from build123d import *

# Parameters (mm, degrees)
P_IDAT_VYSUNUT_M1_DEPTH   = 4.999999888
ODEBRAT_VYSUNUT_M1_DEPTH  = 84.910666461
SKICA3_W                  = 16.00000076
SKICA3_H                  = 5.000002682
P_IDAT_VYSUNUT_M2_DEPTH   = 20
ODEBRAT_VYSUNUT_M3_DEPTH  = 87.116200856
ODEBRAT_VYSUNUT_M4_DEPTH  = 87.116200856
ODEBRAT_VYSUNUT_M5_DEPTH  = 87.116200856
ODEBRAT_VYSUNUT_M6_DEPTH  = 87.116200856
ZKOSEN_1_SIZE             = 4.000000656
ZKOSEN_2_SIZE             = 4.999998957
ZKOSEN_2_SIZE_2           = 4.999999888
ZKOSEN_3_SIZE             = 3.999999976
ZKOSEN_3_SIZE2            = 4.000000587
SKICA11_R                 = 1.7
ODEBRAT_VYSUNUT_M9_DEPTH  = 10
SKICA12_W                 = 16.00000076
SKICA12_H                 = 5.000002682
P_IDAT_VYSUNUT_M3_DEPTH   = 9
SKICA10_R                 = 1.6
SKICA10_R_2               = 1.599999993
ODEBRAT_VYSUNUT_M10_DEPTH = 9


with BuildPart() as part:
    # Skica1 → Přidat vysunutím1 (new body)
    with BuildSketch(Plane.XY.offset(4.999999888)):
        Polygon((45.999998971, 70.000000298), (-29.500000179, 70.000000298), (-29.500000179, 6.8e-07), (9.999999776, 6.8e-07), (45.999998971, 64.999998915), align=None)
    extrude(amount=-P_IDAT_VYSUNUT_M1_DEPTH)

    # Skica2 → Odebrat vysunutím1 (cut, through all)
    with BuildSketch(Plane.XY.offset(4.999999888)):
        Polygon((25.833334774, 59.999998659), (30.000000641, 64.999996523), (30.000000641, 70.000000298), (-29.500000179, 70.000000298), (-29.500000179, 41.000001132), (9.999999776, 41.000001132), align=None)
    extrude(amount=-ODEBRAT_VYSUNUT_M1_DEPTH, mode=Mode.SUBTRACT)

    # Skica3 → Přidat vysunutím2 (add)
    with BuildSketch(Plane.XY.offset(4.999999888)):
        with Locations((37.999999709, 67.499998957)):
            Rectangle(SKICA3_W, SKICA3_H)
    extrude(amount=P_IDAT_VYSUNUT_M2_DEPTH)

    # Skica5 → Odebrat vysunutím3 (cut, through all)
    with BuildSketch(Plane.XY.offset(4.999999888)):
        Polygon((-23.097474128, 4.468092229), (-23.010937497, 4.819194786), (-23.010937497, 5.180804525), (-23.097474128, 5.531907082), (-23.265523836, 5.85209718), (-23.505315185, 6.122766063), (-23.802915588, 6.328184158), (-24.141026661, 6.456412841), (-24.499999359, 6.500000134), (-24.85897392, 6.456412841), (-25.197084993, 6.328184158), (-25.494683534, 6.122766063), (-25.734476745, 5.85209718), (-25.90252459, 5.531907082), (-25.989063084, 5.180804525), (-25.989063084, 4.819194786), (-25.90252459, 4.468092229), (-25.734476745, 4.147903062), (-25.494683534, 3.877233714), (-25.197084993, 3.671815852), (-24.85897392, 3.543587169), (-24.499999359, 3.500000108), (-24.141026661, 3.543587169), (-23.802915588, 3.671815852), (-23.505315185, 3.877233714), (-23.265523836, 4.147903062), align=None)
    extrude(amount=-ODEBRAT_VYSUNUT_M3_DEPTH, mode=Mode.SUBTRACT)

    # Skica6 → Odebrat vysunutím4 (cut, through all)
    with BuildSketch(Plane.XY.offset(4.999999888)):
        Polygon((5.505315959, 3.877233714), (5.802914966, 3.671815852), (6.141026504, 3.543587169), (6.500000134, 3.500000108), (6.858973298, 3.543587169), (7.197084371, 3.671815852), (7.494683843, 3.877233714), (7.734475657, 4.147903062), (7.902524434, 4.468092229), (7.989062928, 4.819194786), (7.989062928, 5.180804525), (7.902524434, 5.531907082), (7.734475657, 5.85209718), (7.494683843, 6.122766063), (7.197084371, 6.328184158), (6.858973298, 6.456412841), (6.500000134, 6.500000134), (6.141026504, 6.456412841), (5.802914966, 6.328184158), (5.505315959, 6.122766063), (5.26552368, 5.85209718), (5.097475369, 5.531907082), (5.010936875, 5.180804525), (5.010936875, 4.819194786), (5.097475369, 4.468092229), (5.26552368, 4.147903062), align=None)
    extrude(amount=-ODEBRAT_VYSUNUT_M4_DEPTH, mode=Mode.SUBTRACT)

    # Skica7 → Odebrat vysunutím5 (cut, through all)
    with BuildSketch(Plane.XY.offset(4.999999888)):
        Polygon((-23.377234116, 35.005312413), (-23.171816021, 35.302914679), (-23.043585941, 35.641025752), (-23.000000045, 35.99999845), (-23.043585941, 36.358974874), (-23.171816021, 36.697082222), (-23.377234116, 36.994680762), (-23.647902533, 37.234473974), (-23.968091235, 37.402521819), (-24.319194257, 37.489064038), (-24.680804461, 37.489064038), (-25.031907484, 37.402521819), (-25.352096185, 37.234473974), (-25.622766465, 36.994680762), (-25.82818456, 36.697082222), (-25.956412777, 36.358974874), (-26.000000536, 35.99999845), (-25.956412777, 35.641025752), (-25.82818456, 35.302914679), (-25.622766465, 35.005312413), (-25.352096185, 34.765522927), (-25.031907484, 34.597471356), (-24.680804461, 34.510936588), (-24.319194257, 34.510936588), (-23.968091235, 34.597471356), (-23.647902533, 34.765522927), align=None)
    extrude(amount=-ODEBRAT_VYSUNUT_M5_DEPTH, mode=Mode.SUBTRACT)

    # Skica8 → Odebrat vysunutím6 (cut, through all)
    with BuildSketch(Plane.XY.offset(4.999999888)):
        Polygon((5.968092475, 34.597471356), (6.319194566, 34.510936588), (6.68080477, 34.510936588), (7.031906862, 34.597471356), (7.35209696, 34.765522927), (7.622765843, 35.005312413), (7.828184403, 35.302914679), (7.956412621, 35.641025752), (8.00000038, 35.99999845), (7.956412621, 36.358974874), (7.828184403, 36.697082222), (7.622765843, 36.994680762), (7.35209696, 37.234473974), (7.031906862, 37.402521819), (6.68080477, 37.489064038), (6.319194566, 37.489064038), (5.968092475, 37.402521819), (5.647902843, 37.234473974), (5.377233494, 36.994680762), (5.171815865, 36.697082222), (5.043587182, 36.358974874), (4.999999888, 35.99999845), (5.043587182, 35.641025752), (5.171815865, 35.302914679), (5.377233494, 35.005312413), (5.647902843, 34.765522927), align=None)
    extrude(amount=-ODEBRAT_VYSUNUT_M6_DEPTH, mode=Mode.SUBTRACT)

    # Zkosení1
    zkosen_1_edges = [part.edges().sort_by_distance(p)[0] for p in [
        (-29.500000179, 41.000001132, 2.499999944),
    ]]
    chamfer(zkosen_1_edges, length=ZKOSEN_1_SIZE)

    # Zkosení2
    # the kernel refuses this chamfer: 4.999999888, 4.999998957 mm, written as the material it adds along each edge
    with BuildSketch(Plane(origin=(58.858412936, 64.999997616, 4.999999888), x_dir=(0, -0.999621916702082, -0.027495884216655726), z_dir=(-1, 0, 0))) as zkosen_2_piece_1_section:
        Polygon((ZKOSEN_2_SIZE * 0.999621916686, ZKOSEN_2_SIZE * 0.0274958842162), (-ZKOSEN_2_SIZE_2 * 0.027495884218, ZKOSEN_2_SIZE_2 * 0.99962191675), (0, 0), align=None)
    zkosen_2_piece_1 = extrude(amount=41.716826979, mode=Mode.PRIVATE)
    zkosen_2_piece_1 = split(zkosen_2_piece_1, bisect_by=Plane(origin=(43.332283636, 60.183290695, 6.69217666), z_dir=(-0.8747913551064548, 0.4844998297533371, 0)), keep=Keep.TOP, mode=Mode.PRIVATE)
    zkosen_2_piece_1 = split(zkosen_2_piece_1, bisect_by=Plane(origin=(32.300745654, 67.760889889, 6.69217666), z_dir=(0.7682212055202173, -0.6401844885570597, 0)), keep=Keep.TOP, mode=Mode.PRIVATE)
    add(zkosen_2_piece_1)

    # Zkosení3
    zkosen_3_edges = [part.edges().sort_by_distance(p)[0] for p in [
        (-29.500000179, 6.8e-07, 2.499999944),
    ]]
    zkosen_3_side = [part.faces().sort_by_distance(p)[0] for p in [
        (-9.750000201, 6.8e-07, 2.499999944),
    ]]
    chamfer(zkosen_3_edges, length=ZKOSEN_3_SIZE, length2=ZKOSEN_3_SIZE2, reference=zkosen_3_side[0])

    # Skica11 → Odebrat vysunutím9 (cut)
    with BuildSketch(Plane(origin=(0, 0, 0), x_dir=(-1, 0, 0), z_dir=(0, 0, -1))):
        with Locations((-6.500000134, 35.99999845)):
            Circle(SKICA11_R)
        with Locations((24.499998894, 35.99999845)):
            Circle(SKICA11_R)
        with Locations((-6.500000134, 4.999999655)):
            Circle(SKICA11_R)
        with Locations((24.499999359, 4.999999655)):
            Circle(SKICA11_R)
    extrude(amount=-ODEBRAT_VYSUNUT_M9_DEPTH, mode=Mode.SUBTRACT)

    # Skica12 → Přidat vysunutím3 (add)
    with BuildSketch(Plane.XY.offset(24.999999888)):
        with Locations((37.999999709, 67.499998957)):
            Rectangle(SKICA12_W, SKICA12_H)
    extrude(amount=P_IDAT_VYSUNUT_M3_DEPTH)

    # Skica10 → Odebrat vysunutím10 (cut)
    with BuildSketch(Plane.XZ.offset(-64.999997616)):
        with Locations(Location((32.999999717, 21.999999776, 0), (0, 0, 270))):
            Circle(SKICA10_R)
        with Locations(Location((42.999999717, 21.999999776, 0), (0, 0, 270))):
            Circle(SKICA10_R_2)
    extrude(amount=-ODEBRAT_VYSUNUT_M10_DEPTH, mode=Mode.SUBTRACT)


solid = part.part
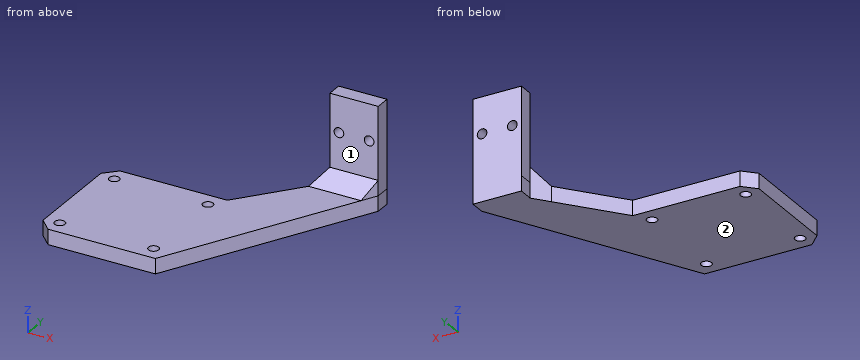
The listing builds one solid part. Answer for the finished solid, in the listing's coordinates (mm). Face numbers are marked on the shaded views. A direction names the side the tool comes from. Round coordinates to 2 decimals unless told otherwise and drop trailing zeros. Write each loop counter-clockwise with the first axis right and the second up, starting at its lowest first coordinate (ties: lowest second). Pieces come first, ordered by that corner, then holes. Notation, with made-up numbers: M 79,42.25 L 86,42.25 A19 cw 86,61.25 Z; hole C -38,80 d2. An arc over 180 degrees is marked long. Write each question's results on one line, items separated by ' | '. Start each with the question number.
(1) The part is cut by section B-B, the plane x = -24.5. Write down the section's boundary in (y, z), and give its area (3 significant figures).
(2) The part is cut by section C-C, the plane z = 4. Write down the section's boundary in (x, y).
(3) For the marked faces 1 and 2, determine the directions among +Z, -Z, +X, -X, +Y, -Y from which every point of the face is accessible in a straight line to the end or side of a thin tool.
(4) Find the intervals of material crossed by line 1 (X direction, y = 67, z = 22); line 2 (Y direction, x = 6.5, z = 2.8); line 3 (Z direction, x = 43, y = 67.55), in increasing order.
(5) The part is cut by section D-D, the plane x = 33. Write down the section's boundary in (y, z).
(6) The part is cut by section A-A, the plane z = 22. Write down the section's boundary in (x, y), and give its area (3 significant figures).
(7) Each of these flat-tipped pins is pushed along its axis until it touches: P1, Ø5.5, axis at y = 66.5, z = 16, coming from the -X side; P2, Ø5.5, axis at x = -4, z = 2.5, coming from the +Y side; P3, Ø2.5, axis at x = 33, z = 22, coming from the +Y side; P4, Ø2, axis at x = 1, y = 11.5, coming from the -Z side. Where does it stop, or does it pass through?
Worked answers:
1) outline: M 0,0 L 3.3,0 L 3.3,5 L 0,5 Z; M 6.7,0 L 34.3,0 L 34.3,5 L 6.7,5 Z; M 37.7,0 L 41,0 L 41,5 L 37.7,5 Z | area: 171 mm²
2) outline: M -29.5,4 L -25.5,0 L 10,0 L 46,65 L 46,70 L 30,70 L 30,65 L 10,41 L -25.5,41 L -29.5,37 Z; hole C -24.5,5 d3.4; hole C -24.5,36 d3.4; hole C 6.5,5 d3.4; hole C 6.5,36 d3.4
3) face 1: +Z, +X, -X, -Y | face 2: -Z, +X, -X, +Y, -Y
4) line 1: x = 30 to 31.4, 34.6 to 41.4, 44.6 to 46 | line 2: y = 0 to 3.3, 6.7 to 34.3, 37.7 to 41 | line 3: z = 0 to 20.4, 23.6 to 34
5) outline: M 41.53,0 L 70,0 L 70,20.4 L 65,20.4 L 65,10 L 60,5 L 41.53,5 Z; M 65,23.6 L 70,23.6 L 70,34 L 65,34 Z
6) outline: M 30,65 L 31.4,65 L 31.4,70 L 30,70 Z; M 34.6,65 L 41.4,65 L 41.4,70 L 34.6,70 Z; M 44.6,65 L 46,65 L 46,70 L 44.6,70 Z | area: 48.0 mm²
7) P1: stops at x = 30 | P2: stops at y = 41 | P3: passes through | P4: stops at z = 0
